from build123d import *

# Parameters (mm, degrees)
F3_DEPTH = 12.5
F5_DEPTH = 12.5
F6_R     = 4
F7_DEPTH = 29.864501
F8_SIZE  = 1.6


with BuildPart() as f1:
    # F0 (on Top) → F1 (revolve)
    with BuildSketch(Plane.XY):
        with BuildLine():
            ThreePointArc((7.104936, -10.962963), (5.675639, -7.871082), (6.558402, -4.581197))
            ThreePointArc((6.558402, -4.581197), (7.970318, 0.6885), (5.675636, 5.63801))
            Line((5.675636, 5.63801), (0, 5.63801))
            Line((0, 5.63801), (0, -10))
            Line((0, -10), (0, -12.361993))
            Line((0, -12.361993), (5.675639, -12.361993))
            ThreePointArc((5.675639, -12.361993), (7.993021, -17.665911), (6.12633, -23.144713))
            ThreePointArc((6.12633, -23.144713), (6.080527, -23.198768), (6.034246, -23.252416))
            ThreePointArc((6.034246, -23.252416), (5.778346, -23.710725), (5.675639, -24.225491))
            Line((5.675639, -24.225491), (7.825808, -24.225491))
            Line((7.825808, -24.225491), (9.398941, -24.225491))
            Line((9.398941, -24.225491), (9.398941, -22.197944))
            ThreePointArc((9.398941, -22.197944), (9.449175, -21.490968), (9.598867, -20.798198))
            ThreePointArc((9.598867, -20.798198), (9.691944, -15.540784), (7.104936, -10.962963))
        make_face()
        with BuildLine():
            ThreePointArc((6.034246, -23.252416), (6.080527, -23.198768), (6.12633, -23.144713))
            ThreePointArc((6.12633, -23.144713), (6.079157, -23.197598), (6.034246, -23.252416))
        make_face()
    revolve(axis=Axis((0, -20.180997, 0), (0, -1, 0)))

    # F2 (on Top) → F3 (cut, symmetric)
    with BuildSketch(Plane.XY):
        with BuildLine():
            Line((-1.5, -17.725491), (-1.5, -24.225491))
            Line((-1.5, -24.225491), (1.5, -24.225491))
            Line((1.5, -24.225491), (1.5, -17.725491))
            ThreePointArc((1.5, -17.725491), (0, -16.225491), (-1.5, -17.725491))
        make_face()
    extrude(amount=F3_DEPTH, both=True, mode=Mode.SUBTRACT)

    # F4 (on Right) → F5 (cut, symmetric)
    with BuildSketch(Plane.YZ):
        with BuildLine():
            Line((-17.682245, 1.5), (-25.682245, 1.5))
            Line((-25.682245, 1.5), (-25.682245, -1.5))
            Line((-25.682245, -1.5), (-17.682245, -1.5))
            ThreePointArc((-17.682245, -1.5), (-16.182245, 0), (-17.682245, 1.5))
        make_face()
    extrude(amount=F5_DEPTH, both=True, mode=Mode.SUBTRACT)

    # F6 (on face) → F7 (cut, through all)
    with BuildSketch(Plane(origin=(0, 5.63801, 0), x_dir=(-1, 0, 0), z_dir=(0, 1, 0))):
        Circle(F6_R)
    extrude(amount=-F7_DEPTH, mode=Mode.SUBTRACT)

    # F8
    f8_edges = [f1.edges().sort_by_distance(p)[0] for p in [
        (4, -12.361993, 0),
    ]]
    chamfer(f8_edges, length=F8_SIZE)


solid = f1.part
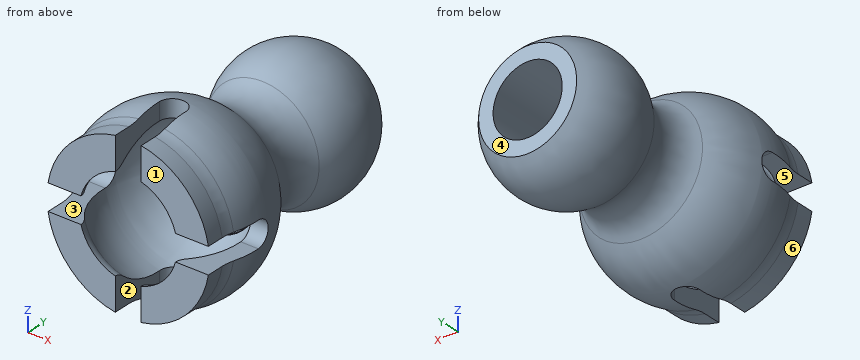
Build history of the part. All positions in model axes, mm. Face numbers are marked on the shaded views. A direction names the side the tool comes from. Round coordinates to 2 decimals unless told otherwise and drop trailing zeros. Write each loop counter-clockwise with the first axis right and the second up, starting at its lowest first coordinate (ties: lowest second). Pieces come first, ordered by that corner, then holes. Notation, with made-up numbers: M -12,79.5 L 24,79.5 A26 ccw 24,117.5 Z; hole C 2.25,64 d1. An arc over 180 degrees is marked long. Answer as a JSON object with one key per item and string values. Group by question number.
(1) Cut at B-B (y = -7.75). Give the cut face in (x, z), and give its area (3 significant figures).
(2) Flat gauge pins, fed straight in: pin 1 (2 mm diameter, centred on x = 7, y = -20.5, fed in from -Z); pin 2 (1.3 mm diameter, centred on y = -20.5, z = -8, fed in from +X); pin 3 (3.5 mm diameter, centred on y = -19.5, z = 8.5, fed in from +X). Where does each tip first touch, or does it go through?
(3) Cut at A-A (y = -18.5). Give the number of separate pieces and of enclosed holes in the cut face, and give its area (3 significant figures).
(4) Which spindle directions (+Z, -Z, +X, -X, +Y, -Y) get a long thin tool onto all of the face, cutting with end or side? Do the marked faces 1, 2 and 3. Say none if no direction does.
(5) Drill centre lines: L1, parallel to Y at x = 4.75, z = 5.25; L2, parallel to Z at x = 0, y = 0.25; L3, parallel to Z at x = 0, y = -5.25. Where is each one in solid material? Low to high.
(6) Mould opens along Z. For the marked faces 4, 5 and 6 say: pulls with the +Z half, pulls with the -Z half, needs draft (parallel to the pull), parting line crosses it, or undercut.
Responses:
{
 "1": {"outline": "C 0,0 d11.33; hole C 0,0 d8", "area": "50.6 mm2"},
 "2": {"pin 1": "stops at z = -7.65", "pin 2": "stops at x = 6.34", "pin 3": "stops at x = 7.25"},
 "3": {"separate pieces": "4", "enclosed holes": "0", "area": "88.9 mm2"},
 "4": {"face 1": "+Z, -Z, +X, -X, -Y", "face 2": "+Z, -Z, -Y", "face 3": "+X, -X, -Y"},
 "5": {"L1": "y = -24.23 to -21.72, -14.28 to -10.94, -3.72 to 3.72", "L2": "z = -8 to -4, 4 to 8", "L3": "z = -6.16 to -4, 4 to 6.16"},
 "6": {"face 4": "needs draft", "face 5": "undercut", "face 6": "pulls with the -Z half"}
}
